Autodesk Inventor part; units mm, degrees
ref_plane "YZ Plane" through (0, 0, 0) normal (1, 0, 0) x (0, 1, 0)
ref_plane "XZ Plane" through (0, 0, 0) normal (0, 1, 0) x (-1, 0, 0)
ref_plane "XY Plane" through (0, 0, 0) normal (0, 0, 1) x (1, 0, 0)
sketch "Sketch2" plane through (0, 0, 0) normal (0, 1, 0) x (-1, 0, 0)
  circle A0 centre (0, 0) radius 16
  circle A1 centre (-150, 0) radius 10
  line L0 (0, 0) -> (-150, 0)
  line L1 (0, 16) -> (-20, 16)
  line L2 (-150, 10) -> (-130, 10)
  spline S0 degree 4 poles (-20, 16) (-33.7807, 16) (-61.342, 16) (-88.658, 10) (-116.2193, 10) (-130, 10) knots 0 0 0 0 0 0.5 1 1 1 1 1
  line L3 (0, 0) -> (0, 16) construction
  line L4 (-150, 0) -> (-150, 10) construction
  line L5 (0, -16) -> (-20, -16)
  line L6 (-150, -10) -> (-130, -10)
  spline S1 degree 4 poles (-20, -16) (-33.7807, -16) (-61.342, -16) (-88.658, -10) (-116.2193, -10) (-130, -10) knots 0 0 0 0 0 0.5 1 1 1 1 1
  line L7 (11.5, 0) -> (-11.5, 0) construction
  dimension "d0" = 32
  dimension "d1" = 20
  dimension "d2" = 150
  dimension "d3" = 20
  dimension "d4" = 20
  dimension "d5" = 23
extrude "Extrusion1" add sketch "Sketch2" along normal blind 5
hole "Hole1" at (-11.5, 0, 0) at (11.5, 0, 0) direction (0, 1, 0) diameter 4.5 end through all
hole "Hole2" at (150, 0, 0) at (0, 0, 0) direction (0, 1, 0) diameter 5.5 end through all
Input: part model. Units: mm. Frame: model coordinates. A direction names the side the tool comes from. Give positions to 0.01 mm unless a question says otherwise; leave off trailing zeros. Order: outer loops, then holes, each group sorted by start corner. A loop starts at its lowest first (then second) coordinate and runs counter-clockwise, first axis right, second up.
Q1. Draft query along X for faces 4 (the cylindrical face through (160, 2, 0)), 5 (the flat face through (10, 2, 16)), 6 (the cylindrical face through (-13.73, 2.54, 0.29)). Return one class per face: +X half, -X half, draft (parallel to the pull), parting line (faces both ways), or undercut.
Checked values:
face 4: +X half
face 5: draft
face 6: undercut
Q2. Contact query for flat-ended pins moving along their axis: pin 1 Ø2.5 at (x, z) = (11.5, 0) entering from +Y; pin 2 Ø1.5 at (x, y) = (140.5, 3.5) entering from -Z. Output: stop coordinate, or through.
Checked values:
pin 1: passes through
pin 2: stops at z = -10
Q3. Section C-C on x = 11.5. Output: boundary loops of the cut face in (y, z).
Checked values:
outline: (0, -16) - (5, -16) - (5, -2.25) - (0, -2.25) - close; (0, 2.25) - (5, 2.25) - (5, 16) - (0, 16) - close
Q4. Ray query, probe 1 along X at (y, z) = (2.6, 0); probe 2 along Z at (x, y) = (0, 1.25); probe 3 along X at (y, z) = (0.3, 1). Return the intervals inside material, ascending.
Checked values:
probe 1: x = -16 to -13.75, -9.25 to -2.75, 2.75 to 9.25, 13.75 to 147.25, 152.75 to 160
probe 2: z = -16 to -2.75, 2.75 to 16
probe 3: x = -15.97 to -13.52, -9.48 to -2.56, 2.56 to 9.48, 13.52 to 147.44, 152.56 to 159.95
Q5. Section A-A on x = -11.5. Output: boundary loops of the cut face in (y, z).
Checked values:
outline: (0, -11.12) - (5, -11.12) - (5, -2.25) - (0, -2.25) - close; (0, 2.25) - (5, 2.25) - (5, 11.12) - (0, 11.12) - close
Q6. Section D-D on z = 8. Output: boundary loops of the cut face in (x, y), and give its area (3 significant figures).
Checked values:
outline: (-13.86, 0) - (156, 0) - (156, 5) - (-13.86, 5) - close
area: 849 mm2
Q7. Set-up query: faces 1 (the cylindrical face through (9.27, 2.54, 0.29)), 2 (the flat face through (140, 2, 10)), 3 (the flat face through (140, 2, -10)). Return all of +Z, -Z, +X, -X, +Y, -Y with unobstructed straight access to the full face (end or side cutting, diameter ignored); none if empty.
Checked values:
face 1: +Y, -Y
face 2: +Z, +X, +Y, -Y
face 3: -Z, +X, +Y, -Y
Q8. Section B-B on y = 1.7. State how many separate pieces and enclosed holes the cut face has, and give its area (3 significant figures).
Checked values:
separate pieces: 1
enclosed holes: 4
area: 4,380 mm2
